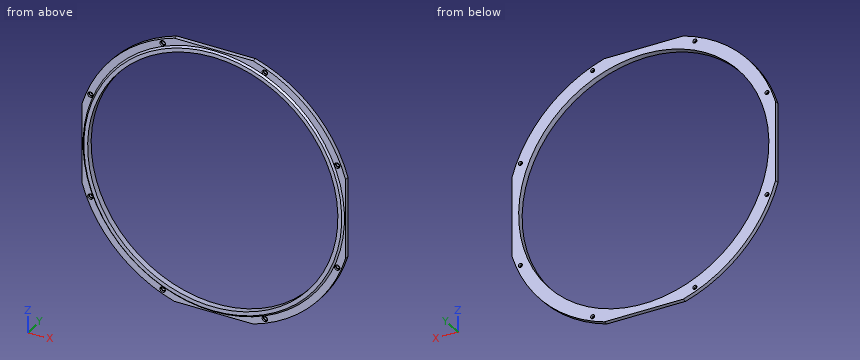
```python
from build123d import *

# Parameters (mm, degrees)
F3_D            = 5.9944
F3_DEPTH        = 25.4
F3_CBORE_D      = 8.001
F3_CBORE_DEPTH  = 2.8448
F3_TIP          = 1.8008994473
F3_COPIES_COUNT = 8
F4_R            = 365.4109378698
F4_W            = 388
F4_H            = 388
F5_DEPTH        = 6.351


# Not quite as in the source:
# - a pattern or mirror of a feature is missing from the dataset's text; its kind, count and spacing are read off the source's solid


with BuildPart() as f1:
    # F0 (on Right) → F1 (revolve)
    with BuildSketch(Plane.YZ):
        Polygon((-8.89, 184.15), (0, 184.15), (0, 202.5), (-6.35, 202.5), (-6.35, 192.34), (-8.89, 189.8), align=None)
    revolve(axis=Axis((0, 77.3353951023, 0), (0, 1, 0)))

    # F3
    with Locations(Plane.XZ.offset(6.35)):
        with Locations((75.1972944597, 181.5423281385)):
            f3 = CounterBoreHole(F3_D / 2, F3_CBORE_D / 2, F3_CBORE_DEPTH, depth=F3_DEPTH)
            with Locations((0, 0, -(F3_DEPTH + F3_TIP / 2))):  # 118° drill point
                Cone(0, F3_D / 2, F3_TIP, mode=Mode.SUBTRACT)

    # F3_copies: F3 ×8 about axis
    f3_copies_axis = Axis((0, 0, 0), (0, 1, 0))
    for i in range(1, F3_COPIES_COUNT):
        add(f3.rotate(f3_copies_axis, i * 360 / F3_COPIES_COUNT), mode=Mode.SUBTRACT)

    # F4 (on face) → F5 (cut, through all)
    with BuildSketch(Plane.XZ.offset(6.35)):
        Circle(F4_R)
        Rectangle(F4_W, F4_H, mode=Mode.SUBTRACT)
    extrude(amount=-F5_DEPTH, mode=Mode.SUBTRACT)


solid = f1.part
```
Input: part model. Units: mm. Frame: model coordinates. Round coordinates to 2 decimals unless told otherwise and drop trailing zeros. Loops run counter-clockwise (first coordinate to the right, second up) from the corner with the lowest first, then second, coordinate; pieces in that order, holes last. Notation, with made-up numbers: M 29,60.5 L 57,60.5 A8 cw 57,67.5 Z; hole C -32.75,-29 d5. An arc over 180 degrees is marked long. Answer in a Markdown table with one row per item. Add a question column.
1. Section A-A (x = 0). Output: boundary loops of the cut face in (y, z).
2. Section C-C (y = -1.75). Give the number of separate pieces and of enclosed holes in the cut face, and give its area (3 significant figures).
3. Section B-B (z = 0). Output: boundary loops of the cut face in (x, y), and give its area (3 significant figures).
4. Ray query, probe 1 along X at (y, z) = (-4.25, -49); probe 2 along X at (y, z) = (-7, -82); probe 3 along Z at (x, y) = (80, -3.25). Return the intervals inside material, ascending.
5. Contact query for flat-ended pins moving along their axis: pin 1 (10 mm diameter, centred on x = 141, z = 146.5, fed in from +Y); pin 2 (9 mm diameter, centred on x = -77, z = -183, fed in from -Y); pin 3 (4 mm diameter, centred on x = -182.5, z = 74, fed in from -Y); pin 4 (1 mm diameter, centred on y = -3, z = 101.5, fed in from -X). Output: stop coordinate, or through.
Values follow:
| question | item | result |
|---|---|---|
| 1 | outline | M -8.89,-189.8 L -6.35,-192.34 L -6.35,-194 L 0,-194 L 0,-184.15 L -8.89,-184.15 Z; M -8.89,184.15 L 0,184.15 L 0,194 L -6.35,194 L -6.35,192.34 L -8.89,189.8 Z |
| 2 | separate pieces | 1 |
| 2 | enclosed holes | 9 |
| 2 | area | 19,400 mm^2 |
| 3 | outline | M -194,-6.35 L -192.34,-6.35 L -189.8,-8.89 L -184.15,-8.89 L -184.15,0 L -194,0 Z; M 184.15,-8.89 L 189.8,-8.89 L 192.34,-6.35 L 194,-6.35 L 194,0 L 184.15,0 Z |
| 3 | area | 160 mm^2 |
| 4 | probe 1 | -194 to -177.51, 177.51 to 194 |
| 4 | probe 2 | -173.27 to -164.89, 164.89 to 173.27 |
| 4 | probe 3 | -186.03 to -165.87, 165.87 to 186.03 |
| 5 | pin 1 | y = 0 |
| 5 | pin 2 | y = -6.35 |
| 5 | pin 3 | y = -3.51 |
| 5 | pin 4 | x = -175.51 |
